Model file for the job. Use its own axes, mm. A direction names the side the tool comes from. Coordinates: 2 decimals unless noted, no trailing zeros. Write each loop counter-clockwise with the first axis right and the second up, starting at its lowest first coordinate (ties: lowest second). Pieces come first, ordered by that corner, then holes.
Q1. Which spindle directions (+Z, -Z, +X, -X, +Y, -Y) get a long thin tool onto all of the face, cutting with end or side? Do faces 5 (the flat face through (75.75, 16, 3)), 6 (the flat face through (83.75, -28, 3)), 7 (the flat face through (20, -30, 3)). Say none if no direction does.
Q2. Drill centre lines: probe 1 along X at (y, z) = (26.5, 2.85); probe 2 along X at (y, z) = (-15.5, 0.75); probe 3 along Y at (x, z) = (-67.5, 4.65). Where is each one in solid material? Low to high.
Q3. Pin check, flat tips, straight feed: P1, Ø3, axis at x = 19, y = -20.5, coming from the -Z side; P2, Ø3, axis at x = 1, z = 1, coming from the +Y side. Stop position of each tip, or through.
Q4. Pull direction X, two halves, no side cores. Call faces 1 (the flat face through (38, -25, 2)), 2 (the flat face through (-1, 0, 0)), 3 (the flat face through (81, 25, 2)), 4 (the flat face through (-100, 0, 3)): released by +X, released by -X, zero draft, split by the parting line, or undercut.
Q5. Band-saw the part on A-A, the plane x = -38.5. Write the cut outline in (y, z), plus the area to 3 significant figures.
from build123d import *

# Parameters (mm, degrees)
SKETCH1_W           = 200
SKETCH1_H           = 50
BOSS_EXTRUDE1_DEPTH = 5
SKETCH2_W           = 5.5
SKETCH2_H           = 2
SKETCH2_W_2         = 3
SKETCH2_H_2         = 12
CUT_EXTRUDE1_DEPTH  = 5
SKETCH3_W           = 16.25
SKETCH3_H           = 5
BOSS_EXTRUDE2_DEPTH = 5


with BuildPart() as part:
    # Sketch1 → Boss-Extrude1 (new body)
    with BuildSketch(Plane.XY):
        Rectangle(SKETCH1_W, SKETCH1_H)
    extrude(amount=BOSS_EXTRUDE1_DEPTH)

    # Sketch2 → Cut-Extrude1 (cut)
    with BuildSketch(Plane.XY.offset(5)):
        with Locations((-77.25, -19)):
            Rectangle(SKETCH2_W, SKETCH2_H)
        with Locations((-77.25, -19)):
            Rectangle(SKETCH2_W_2, SKETCH2_H_2)
        with Locations((0, -19)):
            Rectangle(SKETCH2_W, SKETCH2_H)
        with Locations((0, -19)):
            Rectangle(SKETCH2_W_2, SKETCH2_H_2)
        with Locations((77.25, -19)):
            Rectangle(SKETCH2_W, SKETCH2_H)
        with Locations((77.25, -19)):
            Rectangle(SKETCH2_W_2, SKETCH2_H_2)
    cut_extrude1 = extrude(amount=-CUT_EXTRUDE1_DEPTH, mode=Mode.SUBTRACT)

    # Sketch3 → Boss-Extrude2 (add)
    with BuildSketch(Plane.XY.offset(5)):
        with Locations((-91.875, -27.5)):
            Rectangle(SKETCH3_W, SKETCH3_H)
        with Locations((-19.625, -27.5)):
            Rectangle(SKETCH3_W, SKETCH3_H)
        with Locations((19.625, -27.5)):
            Rectangle(SKETCH3_W, SKETCH3_H)
        with Locations((57.625, -27.5)):
            Rectangle(SKETCH3_W, SKETCH3_H)
        with Locations((91.875, -27.5)):
            Rectangle(SKETCH3_W, SKETCH3_H)
        with Locations((-57.625, -27.5)):
            Rectangle(SKETCH3_W, SKETCH3_H)
    boss_extrude2 = extrude(amount=-BOSS_EXTRUDE2_DEPTH)

    # Mirror1: Cut-Extrude1, Boss-Extrude2 across plane
    add(cut_extrude1.mirror(Plane.ZX), mode=Mode.SUBTRACT)
    add(boss_extrude2.mirror(Plane.ZX))


solid = part.part
Answer sheet:
1. face 5: +Z, -Z, +Y
1. face 6: +Z, -Z, -Y
1. face 7: +Z, -Z, +X, -X, -Y
2. probe 1: x = -100 to -83.75, -65.75 to -49.5, -27.75 to -11.5, 11.5 to 27.75, 49.5 to 65.75, 83.75 to 100
2. probe 2: x = -100 to -78.75, -75.75 to -1.5, 1.5 to 75.75, 78.75 to 100
2. probe 3: y = -25 to 25
3. P1: stops at z = 0
3. P2: stops at y = 25
4. face 1: undercut
4. face 2: zero draft
4. face 3: undercut
4. face 4: released by -X
5. outline: (-25, 0) - (25, 0) - (25, 5) - (-25, 5) - close
5. area: 250 mm2
